Here's how the part is built. I have some questions about the finished solid (model axes, mm). A direction names the side the tool comes from. Give positions to 0.01 mm unless a question says otherwise; leave off trailing zeros. Order: outer loops, then holes, each group sorted by start corner. A loop starts at its lowest first (then second) coordinate and runs counter-clockwise, first axis right, second up.
from build123d import *

# Parameters (mm, degrees)
SKETCH1_W                       = 156
SKETCH1_H                       = 85
SKETCH1_R                       = 17.5
BOSS_EXTRUDE1_DEPTH             = 7.5
SKETCH2_R                       = 21
CUT_EXTRUDE1_DEPTH              = 12
M8_TAPPED_HOLE1_D               = 6.8
M8_TAPPED_HOLE1_DEPTH           = 19.75
M8_TAPPED_HOLE1_TIP             = 2.042926105
M8_TAPPED_HOLE1_ON_FACE_2_D     = 6.8
M8_TAPPED_HOLE1_ON_FACE_2_DEPTH = 19.75
M8_TAPPED_HOLE1_ON_FACE_2_TIP   = 2.042926105
M6_TAPPED_HOLE1_D               = 5
M6_TAPPED_HOLE1_DEPTH           = 15
M6_TAPPED_HOLE1_TIP             = 1.502151548
M6_TAPPED_HOLE1_ON_FACE_2_D     = 5
M6_TAPPED_HOLE1_ON_FACE_2_DEPTH = 15
M6_TAPPED_HOLE1_ON_FACE_2_TIP   = 1.502151548


with BuildPart() as part:
    # Sketch1 → Boss-Extrude1 (new, symmetric)
    with BuildSketch(Plane.XY):
        Rectangle(SKETCH1_W, SKETCH1_H)
        with Locations((-30, 0)):
            Circle(SKETCH1_R, mode=Mode.SUBTRACT)
        with Locations(Location((30, 0, 0), (0, 0, 180))):
            Circle(SKETCH1_R, mode=Mode.SUBTRACT)
    extrude(amount=BOSS_EXTRUDE1_DEPTH, both=True)

    # Sketch2 → Cut-Extrude1 (cut)
    with BuildSketch(Plane.XY.offset(7.5)):
        with Locations((-30, 0)):
            Circle(SKETCH2_R)
        with Locations((30, 0)):
            Circle(SKETCH2_R)
    extrude(amount=-CUT_EXTRUDE1_DEPTH, mode=Mode.SUBTRACT)

    # M8 Tapped Hole1
    with Locations(Plane(origin=(-78, 25, 0), x_dir=(0, 0, -1), z_dir=(-1, 0, 0))):
        with Locations((0, 0), (0, 50)):
            Hole(M8_TAPPED_HOLE1_D / 2, depth=M8_TAPPED_HOLE1_DEPTH)
            with Locations((0, 0, -(M8_TAPPED_HOLE1_DEPTH + M8_TAPPED_HOLE1_TIP / 2))):  # 118° drill point
                Cone(0, M8_TAPPED_HOLE1_D / 2, M8_TAPPED_HOLE1_TIP, mode=Mode.SUBTRACT)

    # M8 Tapped Hole1 on face 2
    with Locations(Plane(origin=(78, 25, 0), x_dir=(0, 0, 1), z_dir=(1, 0, 0))):
        with Locations((0, 0), (0, 50)):
            Hole(M8_TAPPED_HOLE1_ON_FACE_2_D / 2, depth=M8_TAPPED_HOLE1_ON_FACE_2_DEPTH)
            with Locations((0, 0, -(M8_TAPPED_HOLE1_ON_FACE_2_DEPTH + M8_TAPPED_HOLE1_ON_FACE_2_TIP / 2))):  # 118° drill point
                Cone(0, M8_TAPPED_HOLE1_ON_FACE_2_D / 2, M8_TAPPED_HOLE1_ON_FACE_2_TIP, mode=Mode.SUBTRACT)

    # M6 Tapped Hole1
    with Locations(Plane(origin=(-50, -42.5, 0), x_dir=(0, 0, -1), z_dir=(0, -1, 0))):
        with Locations((0, 0), (0, 100)):
            Hole(M6_TAPPED_HOLE1_D / 2, depth=M6_TAPPED_HOLE1_DEPTH)
            with Locations((0, 0, -(M6_TAPPED_HOLE1_DEPTH + M6_TAPPED_HOLE1_TIP / 2))):  # 118° drill point
                Cone(0, M6_TAPPED_HOLE1_D / 2, M6_TAPPED_HOLE1_TIP, mode=Mode.SUBTRACT)

    # M6 Tapped Hole1 on face 2
    with Locations(Plane(origin=(-50, 42.5, 0), x_dir=(0, 0, 1), z_dir=(0, 1, 0))):
        with Locations((0, 0), (0, 100)):
            Hole(M6_TAPPED_HOLE1_ON_FACE_2_D / 2, depth=M6_TAPPED_HOLE1_ON_FACE_2_DEPTH)
            with Locations((0, 0, -(M6_TAPPED_HOLE1_ON_FACE_2_DEPTH + M6_TAPPED_HOLE1_ON_FACE_2_TIP / 2))):  # 118° drill point
                Cone(0, M6_TAPPED_HOLE1_ON_FACE_2_D / 2, M6_TAPPED_HOLE1_ON_FACE_2_TIP, mode=Mode.SUBTRACT)


solid = part.part
Q1. If we section it at A-A on x = -30: List the corners of the cut face in (y, z) for me.
Filled sheet:
outline: (-42.5, -7.5) - (-17.5, -7.5) - (-17.5, -4.5) - (-21, -4.5) - (-21, 7.5) - (-42.5, 7.5) - close; (17.5, -7.5) - (42.5, -7.5) - (42.5, 7.5) - (21, 7.5) - (21, -4.5) - (17.5, -4.5) - close
Q2. If we section it at C-C on z = 5.5: List the corners of the cut face in (x, y) for me.
Filled sheet:
outline: (-78, -42.5) - (78, -42.5) - (78, 42.5) - (-78, 42.5) - close; hole circle Ø42 at (-30, 0); hole circle Ø42 at (30, 0)
Q3. I need wall thicknesses on L1, parallel to X at y = 37.5, z = -0.25; L2, parallel to Y at x = 70, z = -1.75; L3, parallel to Z at x = -72, y = 25. Which ranges of each line are inside material? Lowest first, please.
Filled sheet:
L1: x = -78 to -52.49, -47.51 to 47.51, 52.49 to 78
L2: y = -42.5 to -27.92, -22.08 to 22.08, 27.92 to 42.5
L3: z = -7.5 to -3.4, 3.4 to 7.5
Q4. I'm going to push flat-ended pins straight in: P1, Ø4, axis at x = -50, z = 0, coming from the +Y side; P2, Ø1, axis at x = -12, y = 6, coming from the +Z side; P3, Ø4, axis at x = -50, z = 0, coming from the -Y side. Where does each tip first touch, or does it pass through?
Filled sheet:
P1: stops at y = 27.2
P2: stops at z = -4.5
P3: stops at y = -27.2
Q5. If we section it at D-D on z = -6: List the corners of the cut face in (x, y) for me, plus the area to 3 significant figures.
Filled sheet:
outline: (-78, -42.5) - (78, -42.5) - (78, 42.5) - (-78, 42.5) - close; hole circle Ø35 at (-30, 0); hole circle Ø35 at (30, 0)
area: 11,300 mm2
Q6. Thinking about a two-plate mould opening in Y: for faces 1 (the face through (50, 26, 0)), 2 (the face through (-50, -26, 0)), 3 (the face through (22, 16, -4.5)), which applies, released by +Y, released by -Y, zero draft, split by the parting line, or undercut?
Filled sheet:
face 1: released by +Y
face 2: released by -Y
face 3: undercut
Q7. If we section it at B-B on y = 0: List the corners of the cut face in (x, z) for me, plus the area to 3 significant figures.
Filled sheet:
outline: (-78, -7.5) - (-47.5, -7.5) - (-47.5, -4.5) - (-51, -4.5) - (-51, 7.5) - (-78, 7.5) - close; (-12.5, -7.5) - (12.5, -7.5) - (12.5, -4.5) - (9, -4.5) - (9, 7.5) - (-9, 7.5) - (-9, -4.5) - (-12.5, -4.5) - close; (47.5, -7.5) - (78, -7.5) - (78, 7.5) - (51, 7.5) - (51, -4.5) - (47.5, -4.5) - close
area: 1,120 mm2
Q8. For faces 4 (the face through (-67.99, -28.37, -0.44)), 5 (the face through (50.03, 6.31, 1.58)), 6 (the face through (-52.44, -34.89, -0.54)), which set-ups out of +Z, -Z, +X, -X, +Y, -Y let a thin tool reach every point of the face, with its end or its side?
Filled sheet:
face 4: -X
face 5: +Z
face 6: -Y
